from build123d import *

# Parameters (mm, degrees)
F0_W     = 23.7
F0_H     = 15.7
F1_DEPTH = 12
F2_R     = 2
F3_DEPTH = 3
F4_W     = 20.7
F4_H     = 12.7
F5_DEPTH = 10.5
F6_R     = 2.683106
F6_R_2   = 1.683106
F7_DEPTH = 10


with BuildPart() as f1:
    # F0 (on Top) → F1 (new body)
    with BuildSketch(Plane.XY):
        with Locations((11.85, 7.85)):
            Rectangle(F0_W, F0_H)
    extrude(amount=F1_DEPTH)

    # F2 (on face) → F3 (join)
    with BuildSketch(Plane.XY.offset(12)):
        with Locations((5.35, 11.35)):
            Circle(F2_R)
        with Locations((11.85, 11.35)):
            Circle(F2_R)
        with Locations((18.35, 11.35)):
            Circle(F2_R)
        with Locations((5.35, 4.35)):
            Circle(F2_R)
        with Locations((11.85, 4.35)):
            Circle(F2_R)
        with Locations((18.35, 4.35)):
            Circle(F2_R)
    extrude(amount=F3_DEPTH)

    # F4 (on face) → F5 (cut)
    with BuildSketch(Plane(origin=(0, 0, 0), x_dir=(1, 0, 0), z_dir=(0, 0, -1))):
        with Locations((11.85, -7.85)):
            Rectangle(F4_W, F4_H)
    extrude(amount=-F5_DEPTH, mode=Mode.SUBTRACT)

    # F6 (on face) → F7 (join)
    with BuildSketch(Plane(origin=(0, 0, 10.5), x_dir=(1, 0, 0), z_dir=(0, 0, -1))):
        with Locations((8.612973, -7.835798)):
            Circle(F6_R)
        with Locations((8.612973, -7.835798)):
            Circle(F6_R_2, mode=Mode.SUBTRACT)
        with Locations((15.087027, -7.835798)):
            Circle(F6_R)
        with Locations((15.087027, -7.835798)):
            Circle(F6_R_2, mode=Mode.SUBTRACT)
    extrude(amount=F7_DEPTH)


solid = f1.part
Check sheet for the modelled part. Datum: model origin and axes. Units: mm. A direction names the side the tool comes from. Round coordinates to 2 decimals unless told otherwise and drop trailing zeros. Order: outer loops, then holes, each group sorted by start corner. A loop starts at its lowest first (then second) coordinate and runs counter-clockwise, first axis right, second up.
(1) Scan lines: probe 1 along X at (y, z) = (13, 8.75); probe 2 along Y at (x, z) = (11.75, 4.5); probe 3 along Y at (x, z) = (16.5, 4.75). Record each from-to range of solid material in increasing order.
(2) Access from +Z, -Z, +X, -X, +Y, -Y to the whole of each face (thin tool, end or side, straight path). Record for faces 1 (the flat face through (5, 4, 15)), 2 (the cylindrical face through (6.425, 13.036, 13.479)), 3 (the cylindrical face through (9.851, 10.216, 5.57)).
(3) Cross-section at C-C, the plane y = 11.35. Enter the section's corners in (x, z).
(4) Cross-section at D-D, the plane x = 18.75. Enter the section's corners in (y, z).
(5) Go/stop test with flat-tipped pins: P1, Ø4.5, axis at x = 10, y = 7, coming from the -Z side; P2, Ø4, axis at x = 15.09, y = 7.84, coming from the +Z side; P3, Ø1, axis at x = 15.5, y = 7, coming from the -Z side. Record where each tip stops, or that it passes through.
(6) Cross-section at B-B, the plane x = 5.35. Enter the section's corners in (y, z).
(7) Cross-section at A-A, the plane z = 7.5. Enter the section's corners in (x, y), and give its area (3 significant figures).
Check sheet entries:
1. probe 1: x = 0 to 1.5, 22.2 to 23.7
1. probe 2: y = 0 to 1.5, 14.2 to 15.7
1. probe 3: y = 0 to 1.5, 5.55 to 6.92, 8.75 to 10.12, 14.2 to 15.7
2. face 1: +Z, +X, -X, +Y, -Y
2. face 2: +Z
2. face 3: -Z
3. outline: (0, 0) - (1.5, 0) - (1.5, 10.5) - (22.2, 10.5) - (22.2, 0) - (23.7, 0) - (23.7, 12) - (20.35, 12) - (20.35, 15) - (16.35, 15) - (16.35, 12) - (13.85, 12) - (13.85, 15) - (9.85, 15) - (9.85, 12) - (7.35, 12) - (7.35, 15) - (3.35, 15) - (3.35, 12) - (0, 12) - close
4. outline: (0, 0) - (1.5, 0) - (1.5, 10.5) - (14.2, 10.5) - (14.2, 0) - (15.7, 0) - (15.7, 12) - (13.31, 12) - (13.31, 15) - (9.39, 15) - (9.39, 12) - (6.31, 12) - (6.31, 15) - (2.39, 15) - (2.39, 12) - (0, 12) - close
5. P1: stops at z = 0.5
5. P2: stops at z = 12
5. P3: stops at z = 10.5
6. outline: (0, 0) - (1.5, 0) - (1.5, 10.5) - (14.2, 10.5) - (14.2, 0) - (15.7, 0) - (15.7, 12) - (13.35, 12) - (13.35, 15) - (9.35, 15) - (9.35, 12) - (6.35, 12) - (6.35, 15) - (2.35, 15) - (2.35, 12) - (0, 12) - close
7. outline: (0, 0) - (23.7, 0) - (23.7, 15.7) - (0, 15.7) - close; circle Ø5.37 at (8.61, 7.84); circle Ø5.37 at (15.09, 7.84); hole (1.5, 1.5) - (22.2, 1.5) - (22.2, 14.2) - (1.5, 14.2) - close; hole circle Ø3.37 at (8.61, 7.84); hole circle Ø3.37 at (15.09, 7.84)
7. area: 137 mm2
